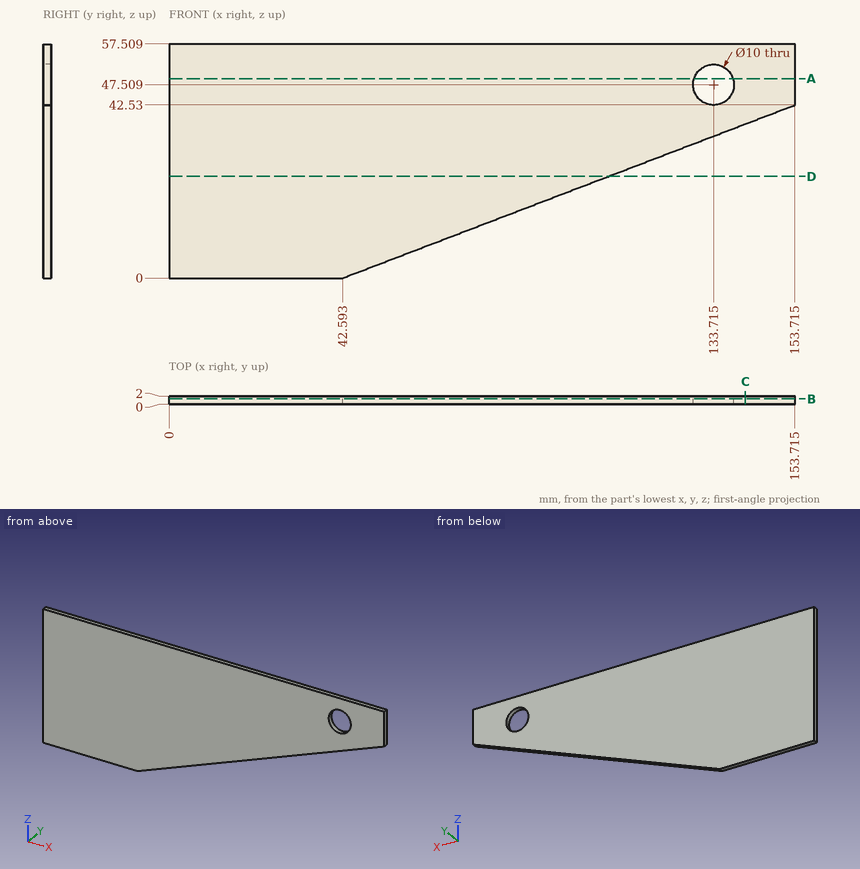
Input: dimensioned drawing with shaded views. Units: mm. Origin: part minimum x, y, z. Round coordinates to 2 decimals unless told otherwise and drop trailing zeros. Order: outer loops, then holes, each group sorted by start corner. A loop starts at its lowest first (then second) coordinate and runs counter-clockwise, first axis right, second up. Notation, with made-up numbers: (-4.75, -3) -> (30.25, -3) arc R26 ccw to (30.25, 19) -> close; hole circle Ø2 at (50, 72.5). An arc over 180 degrees is marked (long way). Put each result on its own line as item: value. Start each with the question number.
Q1. Line query: probe 1 along X at (y, z) = (1.95, 44.5) (1 decimal); probe 2 along Z at (x, y) = (46.5, 1.8) (1 decimal); probe 3 along X at (y, z) = (0.3, 45.5) (1 decimal). Output: solid intervals per line, ascending.
Q2. Section D-D on z = 25. Return the cut outline in (x, y), and give its area (3 significant figures).
Q3. Section B-B on y = 1.35. Return the cut outline in (x, z) (1 decimal), and give its area (3 significant figures).
Q4. Section C-C on x = 141.5. Return the cut outline in (y, z) (1 decimal).
Q5. Section A-A on z = 49. Return the cut outline in (x, y) (1 decimal).
Ans:
1. probe 1: x = 0 to 129.7, 137.7 to 153.7
1. probe 2: z = 1.5 to 57.5
1. probe 3: x = 0 to 129.1, 138.3 to 153.7
2. outline: (0, 0) -> (107.91, 0) -> (107.91, 2) -> (0, 2) -> close
2. area: 216 mm2
3. outline: (0, 0) -> (42.6, 0) -> (153.7, 42.5) -> (153.7, 57.5) -> (0, 57.5) -> close; hole circle Ø10 at (133.7, 47.5)
3. area: 6,400 mm2
4. outline: (0, 37.9) -> (2, 37.9) -> (2, 57.5) -> (0, 57.5) -> close
5. outline: (0, 0) -> (128.9, 0) -> (128.9, 2) -> (0, 2) -> close; (138.5, 0) -> (153.7, 0) -> (153.7, 2) -> (138.5, 2) -> close
